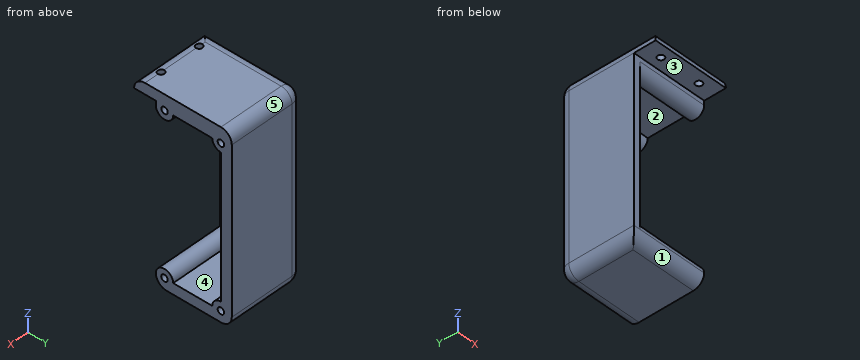
from build123d import *

# Parameters (mm, degrees)
F1_DEPTH     = 17.5
F3_DEPTH     = 3
F5_D         = 3
F5_DEPTH     = 25
F5_TIP       = 0.9012909285
F7_D         = 3
F7_DEPTH     = 25
F7_TIP       = 0.9012909285
F8_T1_DEPTH  = 60
F8_T3_DEPTH  = 42.5
F8_T5_DEPTH  = 75
F8_T7_DEPTH  = 42.5
F8_T9_DEPTH  = 52.5
F8_S13_W     = 5
F8_S13_H     = 5
F8_T14_DEPTH = 5
F8_S19_W     = 5
F8_S19_H     = 5
F8_T20_DEPTH = 5


# Not quite as in the source:
# - a fillet or chamfer that OpenCascade refuses, or shapes differently, is made with other operations: its cross-section is extruded or revolved along the edge and cut away or added


with BuildPart() as f1:
    # F0 (on Right) → F1 (new body, symmetric)
    with BuildSketch(Plane.YZ):
        Polygon((-2.2390836586, 4.4176964641), (-2.2390836586, -0.5823035359), (7.7609163414, -0.5823035359), (7.7609163414, -2.5823035359), (15.7609163414, -2.5823035359), (33.7609163414, -2.5823035359), (37.7609163414, -2.5823035359), (37.7609163414, -6.5823035359), (37.7609163414, -71.5823035359), (37.7609163414, -75.5823035359), (33.7609163414, -75.5823035359), (15.7609163414, -75.5823035359), (7.7609163414, -75.5823035359), (7.7609163414, -80.5823035359), (42.7609163414, -80.5823035359), (42.7609163414, 4.4176964641), align=None)
        with BuildLine():
            Line((15.7609163414, -2.5823035359), (7.7609163414, -2.5823035359))
            ThreePointArc((7.7609163414, -2.5823035359), (11.7609163414, -6.5823035359), (15.7609163414, -2.5823035359))
        make_face()
        with BuildLine():
            Line((37.7609163414, -2.5823035359), (33.7609163414, -2.5823035359))
            ThreePointArc((33.7609163414, -2.5823035359), (34.9324892166, -5.4107306607), (37.7609163414, -6.5823035359))
            Line((37.7609163414, -6.5823035359), (37.7609163414, -2.5823035359))
        make_face()
        with BuildLine():
            ThreePointArc((15.7609163414, -75.5823035359), (11.7609163414, -71.5823035359), (7.7609163414, -75.5823035359))
            Line((7.7609163414, -75.5823035359), (15.7609163414, -75.5823035359))
        make_face()
        with BuildLine():
            Line((37.7609163414, -75.5823035359), (37.7609163414, -71.5823035359))
            ThreePointArc((37.7609163414, -71.5823035359), (34.9324892166, -72.7538764112), (33.7609163414, -75.5823035359))
            Line((33.7609163414, -75.5823035359), (37.7609163414, -75.5823035359))
        make_face()
    extrude(amount=F1_DEPTH, both=True)

    # F2 (on face) → F3 (join)
    with BuildSketch(Plane(origin=(-17.5, 0, 0), x_dir=(0, -1, 0), z_dir=(-1, 0, 0))):
        with BuildLine():
            Line((-7.7609163414, -75.5823035359), (-7.7609163414, -2.5823035359))
            ThreePointArc((-7.7609163414, -2.5823035359), (-11.7609163414, -6.5823035359), (-15.7609163414, -2.5823035359))
            Line((-15.7609163414, -2.5823035359), (-33.7609163414, -2.5823035359))
            ThreePointArc((-33.7609163414, -2.5823035359), (-34.9324892166, -5.4107306607), (-37.7609163414, -6.5823035359))
            Line((-37.7609163414, -6.5823035359), (-37.7609163414, -71.5823035359))
            ThreePointArc((-37.7609163414, -71.5823035359), (-34.9324892166, -72.7538764112), (-33.7609163414, -75.5823035359))
            Line((-33.7609163414, -75.5823035359), (-15.7609163414, -75.5823035359))
            ThreePointArc((-15.7609163414, -75.5823035359), (-11.7609163414, -71.5823035359), (-7.7609163414, -75.5823035359))
        make_face()
    extrude(amount=-F3_DEPTH)

    # F5
    with Locations(Plane.YZ.offset(17.5)):
        with Locations((11.7609163414, -2.5823035359), (37.7609163414, -2.5823035359), (37.7609163414, -75.5823035359), (11.7609163414, -75.5823035359)):
            Hole(F5_D / 2, depth=F5_DEPTH)
            with Locations((0, 0, -(F5_DEPTH + F5_TIP / 2))):  # 118° drill point
                Cone(0, F5_D / 2, F5_TIP, mode=Mode.SUBTRACT)

    # F7
    with Locations(Plane.XY.offset(4.4176964641)):
        with Locations((-9.5, 2.7609163414), (9.5, 2.7609163414)):
            Hole(F7_D / 2, depth=F7_DEPTH)
            with Locations((0, 0, -(F7_DEPTH + F7_TIP / 2))):  # 118° drill point
                Cone(0, F7_D / 2, F7_TIP, mode=Mode.SUBTRACT)

    # F8: fillet of radius 5 on 7 edges, made by hand

    # F8_s2 → F8_t1 (cut)
    with BuildSketch(Plane.YZ.offset(-30)):
        with BuildLine():
            ThreePointArc((2.7609163414, 4.4176964641), (-0.7746175645, 2.95323037), (-2.2390836586, -0.5823035359))
            Line((-2.2390836586, -0.5823035359), (-2.2390836586, 4.4176964641))
            Line((-2.2390836586, 4.4176964641), (2.7609163414, 4.4176964641))
        make_face()
        with BuildLine():
            ThreePointArc((7.7609163414, -75.5823035359), (9.2253824355, -79.1178374419), (12.7609163414, -80.5823035359))
            Line((12.7609163414, -80.5823035359), (7.7609163414, -80.5823035359))
            Line((7.7609163414, -80.5823035359), (7.7609163414, -75.5823035359))
        make_face()
    extrude(amount=F8_T1_DEPTH, mode=Mode.SUBTRACT)

    # F8_s4 → F8_t3 (cut)
    with BuildSketch(Plane.YZ.offset(-12.5)):
        with BuildLine():
            ThreePointArc((42.7609163414, -0.5823035359), (41.2964502473, 2.95323037), (37.7609163414, 4.4176964641))
            Line((37.7609163414, 4.4176964641), (42.7609163414, 4.4176964641))
            Line((42.7609163414, 4.4176964641), (42.7609163414, -0.5823035359))
        make_face()
        with BuildLine():
            ThreePointArc((37.7609163414, -80.5823035359), (41.2964502473, -79.1178374419), (42.7609163414, -75.5823035359))
            Line((42.7609163414, -75.5823035359), (42.7609163414, -80.5823035359))
            Line((42.7609163414, -80.5823035359), (37.7609163414, -80.5823035359))
        make_face()
    extrude(amount=F8_T3_DEPTH, mode=Mode.SUBTRACT)

    # F8_s6 → F8_t5 (cut)
    with BuildSketch(Plane.XY.offset(-75.5823035359)):
        with BuildLine():
            ThreePointArc((-17.5, 37.7609163414), (-16.0355339059, 41.2964502473), (-12.5, 42.7609163414))
            Line((-12.5, 42.7609163414), (-17.5, 42.7609163414))
            Line((-17.5, 42.7609163414), (-17.5, 37.7609163414))
        make_face()
    extrude(amount=F8_T5_DEPTH, mode=Mode.SUBTRACT)

    # F8_s8 → F8_t7 (cut)
    with BuildSketch(Plane.XZ.offset(-37.7609163414)):
        with BuildLine():
            ThreePointArc((-12.5, -80.5823035359), (-16.0355339059, -79.1178374419), (-17.5, -75.5823035359))
            Line((-17.5, -75.5823035359), (-17.5, -80.5823035359))
            Line((-17.5, -80.5823035359), (-12.5, -80.5823035359))
        make_face()
    extrude(amount=F8_T7_DEPTH, mode=Mode.SUBTRACT)

    # F8_s10 → F8_t9 (cut)
    with BuildSketch(Plane.XZ.offset(-37.7609163414)):
        with BuildLine():
            ThreePointArc((-17.5, -0.5823035359), (-16.0355339059, 2.95323037), (-12.5, 4.4176964641))
            Line((-12.5, 4.4176964641), (-17.5, 4.4176964641))
            Line((-17.5, 4.4176964641), (-17.5, -0.5823035359))
        make_face()
    extrude(amount=F8_T9_DEPTH, mode=Mode.SUBTRACT)


with BuildPart() as f8_tool12:
    # F8_s13 → F8_t14 (new body)
    with BuildSketch(Plane.XZ.offset(-37.7609163414)):
        with Locations((-15, 1.9176964641)):
            Rectangle(F8_S13_W, F8_S13_H)
    extrude(amount=-F8_T14_DEPTH)

    # F8_s15 → F8_t16 (revolve, cut)
    with BuildSketch(Plane(origin=(-12.5, 37.7609163414, -0.5823035359), x_dir=(0.7071067812, 0, -0.7071067812), z_dir=(0.7071067812, 0, 0.7071067812))):
        with BuildLine():
            ThreePointArc((0, -5), (5, 0), (0, 5))
            Line((0, 5), (0, -5))
        make_face()
    revolve(axis=Axis((-12.5, 37.7609163414, -0.5823035359), (0, 1, 0)), mode=Mode.SUBTRACT)


with BuildPart() as f1_1:
    add(f1.part)

    # F8_t11: cut F8_tool12
    add(f8_tool12.part, mode=Mode.SUBTRACT)


with BuildPart() as f8_tool18:
    # F8_s19 → F8_t20 (new body)
    with BuildSketch(Plane.XZ.offset(-37.7609163414)):
        with Locations((-15, -78.0823035359)):
            Rectangle(F8_S19_W, F8_S19_H)
    extrude(amount=-F8_T20_DEPTH)

    # F8_s21 → F8_t22 (revolve, cut)
    with BuildSketch(Plane(origin=(-12.5, 37.7609163414, -75.5823035359), x_dir=(0.7071067812, 0, 0.7071067812), z_dir=(-0.7071067812, 0, 0.7071067812))):
        with BuildLine():
            ThreePointArc((0, -5), (5, 0), (0, 5))
            Line((0, 5), (0, -5))
        make_face()
    revolve(axis=Axis((-12.5, 37.7609163414, -75.5823035359), (0, 1, 0)), mode=Mode.SUBTRACT)


with BuildPart() as f1_2:
    add(f1_1.part)

    # F8_t17: cut F8_tool18
    add(f8_tool18.part, mode=Mode.SUBTRACT)


solid = f1_2.part
Work out the finished part from the listing and answer in its coordinate system (mm). Face numbers are marked on the shaded views. A direction names the side the tool comes from. Coordinates: 2 decimals unless noted, no trailing zeros. Loops run counter-clockwise (first coordinate to the right, second up) from the corner with the lowest first, then second, coordinate; pieces in that order, holes last. Notation, with made-up numbers: (-14, 19) -> (-2, 19) arc R10 cw to (-2, 34) -> close; hole circle Ø1 at (60.5, -39). An arc over 180 degrees is marked (long way). Answer as CSV lines item,"result".
1) The part is cut by section D-D (z = -66.5). Give the vertices of the cut face in (x, y).
A:
outline,"(-17.5, 7.76) -> (-14.5, 7.76) -> (-14.5, 37.76) -> (17.5, 37.76) -> (17.5, 42.76) -> (-12.5, 42.76) arc R5 ccw to (-17.5, 37.76) -> close"
2) The part is cut by section B-B (x = 9.5). Give the vertices of the cut face in (y, z).
A:
outline,"(-2.24, -0.58) -> (1.26, -0.58) -> (1.26, 4.19) arc R5 ccw to start; (4.26, -0.58) -> (7.76, -0.58) -> (7.76, -2.58) arc R4 ccw to (15.76, -2.58) -> (33.76, -2.58) arc R4 ccw to (37.76, -6.58) -> (37.76, -71.58) arc R4 ccw to (33.76, -75.58) -> (15.76, -75.58) arc R4 ccw to (7.76, -75.58) arc R5 ccw to (12.76, -80.58) -> (37.76, -80.58) arc R5 ccw to (42.76, -75.58) -> (42.76, -0.58) arc R5 ccw to (37.76, 4.42) -> (4.26, 4.42) -> close; hole circle Ø3 at (11.76, -75.58); hole circle Ø3 at (11.76, -2.58); hole circle Ø3 at (37.76, -75.58); hole circle Ø3 at (37.76, -2.58)"
3) Straight lines are drawn through the part: probe 1 along Z at (x, y) = (15, 17); probe 2 along Y at (x, z) = (-3, -57.5); probe 3 along X at (y, z) = (13.5, -53.5). For each, find the intervals that lie inside material, in ascending order.
A:
probe 1,"z = -80.58 to -75.58, -2.58 to 4.42"
probe 2,"y = 37.76 to 42.76"
probe 3,"x = -17.5 to -14.5"
4) The part is cut by section A-A (x = -6.5). Give the vertices of the cut face in (y, z), and give its area (3 significant figures).
A:
outline,"(-2.24, -0.58) -> (7.76, -0.58) -> (7.76, -2.58) arc R4 ccw to (15.76, -2.58) -> (33.76, -2.58) arc R4 ccw to (37.76, -6.58) -> (37.76, -71.58) arc R4 ccw to (33.76, -75.58) -> (15.76, -75.58) arc R4 ccw to (7.76, -75.58) arc R5 ccw to (12.76, -80.58) -> (37.76, -80.58) arc R5 ccw to (42.76, -75.58) -> (42.76, -0.58) arc R5 ccw to (37.76, 4.42) -> (2.76, 4.42) arc R5 ccw to start; hole circle Ø3 at (11.76, -75.58); hole circle Ø3 at (11.76, -2.58); hole circle Ø3 at (37.76, -75.58); hole circle Ø3 at (37.76, -2.58)"
area,"861 mm²"
5) Flat-ended cylindrical pins translate along their axes: pin 1 (6 mm diameter, centred on x = 2, z = -71, fed in from -Y); pin 2 (2.5 mm diameter, centred on y = 37.76, z = -75.58, fed in from +X); pin 3 (9 mm diameter, centred on y = 20, z = -50, fed in from +X); pin 4 (1.5 mm diameter, centred on y = 6.5, z = -19, fed in from -X) (1 decimal). Find the tip coordinate at first contact, or state that the pin passes through.
A:
pin 1,"stops at y = 8.09"
pin 2,"stops at x = -7.65"
pin 3,"stops at x = -14.5"
pin 4,"passes through"
6) The part is cut by section C-C (y = 17). Give the vertices of the cut face in (x, z), and give its area (3 significant figures).
A:
outline,"(-17.5, -75.58) arc R5 ccw to (-12.5, -80.58) -> (17.5, -80.58) -> (17.5, -75.58) -> (-14.5, -75.58) -> (-14.5, -2.58) -> (17.5, -2.58) -> (17.5, 4.42) -> (-12.5, 4.42) arc R5 ccw to (-17.5, -0.58) -> close"
area,"628 mm²"
7) For the marked faces 1 and 2, determine the directions among +Z, -Z, +X, -X, +Y, -Y from which every point of the face is accessible in a straight line to the end or side of a thin tool.
A:
face 1,"-Z, +X, -X, -Y"
face 2,"+X"
8) For a pull along Y with two mould halves and no side action, classify the marked faces 3, 4 and 5 as released by +Y, released by -Y, zero draft, split by the parting line, or undercut.
A:
face 3,"zero draft"
face 4,"undercut"
face 5,"released by +Y"
